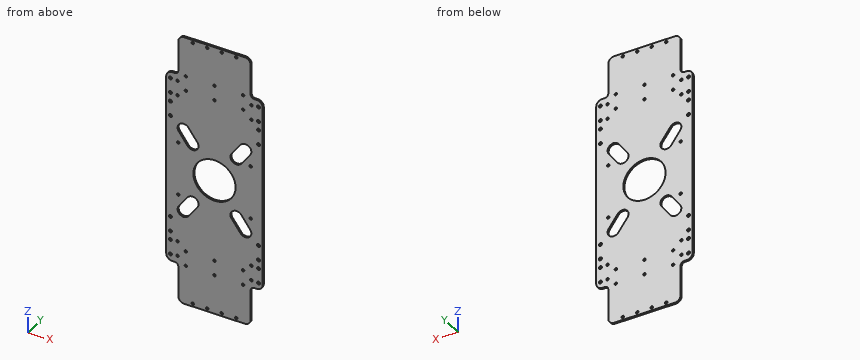
from build123d import *

# Parameters (mm, degrees)
EXTRUDE_1_DEPTH     = 3
SKETCH_2_R          = 2.6
SKETCH_2_R_2        = 35
SKETCH_2_R_3        = 2.1
CUT_EXTRUDE_1_DEPTH = 10
CUT_EXTRUDE_2_DEPTH = 10
SKETCH_8_R          = 2.1
CUT_EXTRUDE_6_DEPTH = 10
SKETCH_9_R          = 2.1
CUT_EXTRUDE_7_DEPTH = 10


with BuildPart() as part:
    # 草图1 → 凸台-拉伸1 (new body)
    with BuildSketch(Plane(origin=(0, 0, 0), x_dir=(1, 0, 0), z_dir=(0, 1, 0))):
        with BuildLine():
            Line((165, -108), (161, -108))
            ThreePointArc((161, -108), (156.757359313, -109.757359313), (155, -114))
            Line((155, -114), (155, -165))
            ThreePointArc((155, -165), (152.071067812, -172.071067812), (145, -175))
            Line((145, -175), (45, -175))
            ThreePointArc((45, -175), (37.928932188, -172.071067812), (35, -165))
            Line((35, -165), (35, -114))
            ThreePointArc((35, -114), (33.242640687, -109.757359313), (29, -108))
            Line((29, -108), (25, -108))
            ThreePointArc((25, -108), (17.928932188, -105.071067812), (15, -98))
            Line((15, -98), (15, -25))
            Line((15, -25), (15, 135))
            Line((15, 135), (15, 208))
            ThreePointArc((15, 208), (17.928932188, 215.071067812), (25, 218))
            Line((25, 218), (29, 218))
            ThreePointArc((29, 218), (33.242640687, 219.757359313), (35, 224))
            Line((35, 224), (35, 275))
            ThreePointArc((35, 275), (37.928932188, 282.071067812), (45, 285))
            Line((45, 285), (145, 285))
            ThreePointArc((145, 285), (152.071067812, 282.071067812), (155, 275))
            Line((155, 275), (155, 224))
            ThreePointArc((155, 224), (156.757359313, 219.757359313), (161, 218))
            Line((161, 218), (165, 218))
            ThreePointArc((165, 218), (172.071067812, 215.071067812), (175, 208))
            Line((175, 208), (175, 135))
            Line((175, 135), (175, -25))
            Line((175, -25), (175, -98))
            ThreePointArc((175, -98), (172.071067812, -105.071067812), (165, -108))
        make_face()
    extrude(amount=EXTRUDE_1_DEPTH)

    # 草图2 → 切除-拉伸1 (cut)
    with BuildSketch(Plane.XZ):
        with Locations(Location((168.1, 97, 0), (0, 0, 270))):
            Circle(SKETCH_2_R)
        with Locations(Location((168.1, 72, 0), (0, 0, 270))):
            Circle(SKETCH_2_R)
        with Locations(Location((168.1, 57, 0), (0, 0, 270))):
            Circle(SKETCH_2_R)
        with Locations(Location((168.1, 32, 0), (0, 0, 270))):
            Circle(SKETCH_2_R)
        with Locations(Location((95, -55, 0), (0, 0, 270))):
            Circle(SKETCH_2_R_2)
        with Locations(Location((59, 170, 0), (0, 0, 270))):
            Circle(SKETCH_2_R_3)
        with Locations(Location((83, 170, 0), (0, 0, 270))):
            Circle(SKETCH_2_R_3)
        with Locations(Location((107, 170, 0), (0, 0, 270))):
            Circle(SKETCH_2_R_3)
        with Locations(Location((131, 170, 0), (0, 0, 270))):
            Circle(SKETCH_2_R_3)
        with Locations(Location((131, -280, 0), (0, 0, 270))):
            Circle(SKETCH_2_R_3)
        with Locations(Location((107, -280, 0), (0, 0, 270))):
            Circle(SKETCH_2_R_3)
        with Locations(Location((83, -280, 0), (0, 0, 270))):
            Circle(SKETCH_2_R_3)
        with Locations(Location((59, -280, 0), (0, 0, 270))):
            Circle(SKETCH_2_R_3)
        with Locations(Location((142.5, 108.632151192, 0), (0, 0, 270))):
            Circle(SKETCH_2_R_3)
        with Locations(Location((142.5, 83.632151192, 0), (0, 0, 270))):
            Circle(SKETCH_2_R_3)
        with Locations(Location((95, 83.632151192, 0), (0, 0, 270))):
            Circle(SKETCH_2_R_3)
        with Locations(Location((95, 108.632151192, 0), (0, 0, 270))):
            Circle(SKETCH_2_R_3)
        with Locations(Location((47.5, 83.632151192, 0), (0, 0, 270))):
            Circle(SKETCH_2_R_3)
        with Locations(Location((47.5, 108.632151192, 0), (0, 0, 270))):
            Circle(SKETCH_2_R_3)
        with Locations(Location((47.5, -218.632151192, 0), (0, 0, 270))):
            Circle(SKETCH_2_R_3)
        with Locations(Location((47.5, -193.632151192, 0), (0, 0, 270))):
            Circle(SKETCH_2_R_3)
        with Locations(Location((95, -218.632151192, 0), (0, 0, 270))):
            Circle(SKETCH_2_R_3)
        with Locations(Location((95, -193.632151192, 0), (0, 0, 270))):
            Circle(SKETCH_2_R_3)
        with Locations(Location((142.5, -193.632151192, 0), (0, 0, 270))):
            Circle(SKETCH_2_R_3)
        with Locations(Location((142.5, -218.632151192, 0), (0, 0, 270))):
            Circle(SKETCH_2_R_3)
        with Locations(Location((21.9, 32, 0), (0, 0, 270))):
            Circle(SKETCH_2_R)
        with Locations(Location((21.9, 57, 0), (0, 0, 270))):
            Circle(SKETCH_2_R)
        with Locations(Location((21.9, 72, 0), (0, 0, 270))):
            Circle(SKETCH_2_R)
        with Locations(Location((21.9, 97, 0), (0, 0, 270))):
            Circle(SKETCH_2_R)
        with Locations(Location((21.9, -207, 0), (0, 0, 270))):
            Circle(SKETCH_2_R)
        with Locations(Location((21.9, -182, 0), (0, 0, 270))):
            Circle(SKETCH_2_R)
        with Locations(Location((21.9, -167, 0), (0, 0, 270))):
            Circle(SKETCH_2_R)
        with Locations(Location((21.9, -142, 0), (0, 0, 270))):
            Circle(SKETCH_2_R)
        with Locations(Location((168.1, -142, 0), (0, 0, 270))):
            Circle(SKETCH_2_R)
        with Locations(Location((168.1, -167, 0), (0, 0, 270))):
            Circle(SKETCH_2_R)
        with Locations(Location((168.1, -182, 0), (0, 0, 270))):
            Circle(SKETCH_2_R)
        with Locations(Location((168.1, -207, 0), (0, 0, 270))):
            Circle(SKETCH_2_R)
    extrude(amount=-CUT_EXTRUDE_1_DEPTH, mode=Mode.SUBTRACT)

    # 草图3 → 切除-拉伸2 (cut)
    with BuildSketch(Plane.XZ):
        with BuildLine():
            Line((35.772513107, -119.506625988), (50.467144414, -99.281201128))
            ThreePointArc((50.467144414, -99.281201128), (64.435166881, -97.068883707), (66.647484302, -111.036906174))
            Line((66.647484302, -111.036906174), (51.952852994, -131.262331034))
            ThreePointArc((51.952852994, -131.262331034), (37.984830528, -133.474648454), (35.772513107, -119.506625988))
        make_face()
        with BuildLine():
            Line((51.952852994, 21.262331034), (66.647484302, 1.036906174))
            ThreePointArc((66.647484302, 1.036906174), (64.435166881, -12.931116293), (50.467144414, -10.718798872))
            Line((50.467144414, -10.718798872), (35.772513107, 9.506625988))
            ThreePointArc((35.772513107, 9.506625988), (37.984830528, 23.474648454), (51.952852994, 21.262331034))
        make_face()
        with BuildLine():
            Line((154.227486893, 9.506625988), (139.532855586, -10.718798872))
            ThreePointArc((139.532855586, -10.718798872), (125.564833119, -12.931116293), (123.352515698, 1.036906174))
            Line((123.352515698, 1.036906174), (138.047147006, 21.262331034))
            ThreePointArc((138.047147006, 21.262331034), (152.015169472, 23.474648454), (154.227486893, 9.506625988))
        make_face()
        with BuildLine():
            Line((138.047147006, -131.262331034), (123.352515698, -111.036906174))
            ThreePointArc((123.352515698, -111.036906174), (125.564833119, -97.068883707), (139.532855586, -99.281201128))
            Line((139.532855586, -99.281201128), (154.227486893, -119.506625988))
            ThreePointArc((154.227486893, -119.506625988), (152.015169472, -133.474648454), (138.047147006, -131.262331034))
        make_face()
    extrude(amount=-CUT_EXTRUDE_2_DEPTH, mode=Mode.SUBTRACT)

    # 草图8 → 切除-拉伸6 (cut)
    with BuildSketch(Plane(origin=(0, 3, 0), x_dir=(1, 0, 0), z_dir=(0, 1, 0))):
        with Locations(Location((155, 10, 0), (0, 0, 270))):
            Circle(SKETCH_8_R)
        with Locations(Location((155, 100, 0), (0, 0, 90))):
            Circle(SKETCH_8_R)
        with Locations(Location((35, 10, 0), (0, 0, 90))):
            Circle(SKETCH_8_R)
        with Locations(Location((35, 100, 0), (0, 0, 270))):
            Circle(SKETCH_8_R)
    extrude(amount=-CUT_EXTRUDE_6_DEPTH, mode=Mode.SUBTRACT)

    # 草图9 → 切除-拉伸7 (cut)
    with BuildSketch(Plane(origin=(0, 3, 0), x_dir=(1, 0, 0), z_dir=(0, 1, 0))):
        with Locations(Location((156.2, -71, 0), (0, 0, 270))):
            Circle(SKETCH_9_R)
        with Locations(Location((156.2, -96, 0), (0, 0, 270))):
            Circle(SKETCH_9_R)
        with Locations(Location((33.8, -96, 0), (0, 0, 90))):
            Circle(SKETCH_9_R)
        with Locations(Location((33.8, -71, 0), (0, 0, 90))):
            Circle(SKETCH_9_R)
        with Locations(Location((156.2, 181, 0), (0, 0, 90))):
            Circle(SKETCH_9_R)
        with Locations(Location((156.2, 206, 0), (0, 0, 90))):
            Circle(SKETCH_9_R)
        with Locations(Location((33.8, 181, 0), (0, 0, 270))):
            Circle(SKETCH_9_R)
        with Locations(Location((33.8, 206, 0), (0, 0, 270))):
            Circle(SKETCH_9_R)
    extrude(amount=-CUT_EXTRUDE_7_DEPTH, mode=Mode.SUBTRACT)


solid = part.part
For this review, take the finished solid that the model builds, in its own axes (mm). Give positions to 0.01 mm unless a question says otherwise; leave off trailing zeros. Order: outer loops, then holes, each group sorted by start corner. A loop starts at its lowest first (then second) coordinate and runs counter-clockwise, first axis right, second up. Notation, with made-up numbers: (74, -32.5) -> (93, -32.5) arc R30 ccw to (93, -0.5) -> close; hole circle Ø7 at (-26, 24). An arc over 180 degrees is marked (long way). Write item = value, one per line.
1) We need section A-A, the plane z = -55. Give the boundary of the cut face in (x, y).
Findings:
outline = (15, 0) -> (60, 0) -> (60, 3) -> (15, 3) -> close; (130, 0) -> (175, 0) -> (175, 3) -> (130, 3) -> close
2) We need section C-C, the plane y = 1.75. Count the separate pieces of the cut face and the enclosed holes in it, and give its area (3 significant figures).
Findings:
separate_pieces = 1
enclosed_holes = 53
area = 60,200 mm^2
3) We need section B-B, the plane x = 101. Give the boundary of the cut face in (y, z), and give its area (3 significant figures).
Findings:
outline = (0, -285) -> (3, -285) -> (3, -89.48) -> (0, -89.48) -> close; (0, -20.52) -> (3, -20.52) -> (3, 175) -> (0, 175) -> close
area = 1,170 mm^2
4) Insertion check: pin 1 (4 mm diameter, centred on x = 35, z = -10, fed in from -Y); pin 2 (2 mm diameter, centred on x = 52.5, z = -42, fed in from -Y). Each pin has a flat end and moves straight along its axis. Give the tip position at first contact, or say it passes through.
Findings:
pin_1 = through
pin_2 = 0
5) To check wall thickness, follow L1, parallel to X at y = 2.1, z = 96; L2, parallel to X at y = 1.2, z = 6; L3, parallel to X at y = 2.45, z = 170. State the ranges of each line that lie inside material, in increasing order. Write a range as from..to.
Findings:
L1 = 15..19.5, 24.3..31.7, 35.9..154.1, 158.3..165.7, 170.5..175
L2 = 15..38.32, 63.04..126.96, 151.68..175
L3 = 36.34..56.9, 61.1..80.9, 85.1..104.9, 109.1..128.9, 133.1..153.66
